Could you check a few things on this model? Use its own coordinates, in mm. Face numbers are marked on the shaded views. A direction names the side the tool comes from. Round coordinates to 2 decimals unless told otherwise and drop trailing zeros. Order: outer loops, then holes, each group sorted by start corner. A loop starts at its lowest first (then second) coordinate and runs counter-clockwise, first axis right, second up. Notation, with made-up numbers: (5, -38.5) - (28, -38.5) arc R23 cw to (28, 0.5) - close; hole circle Ø3 at (-24, 75.25). An arc over 180 degrees is marked (long way). Use one line per item in the form item = value.
from build123d import *

# Parameters (mm, degrees)
TABAN_FLAN_1_DEPTH       = 400
M5_DI_LI_DELIK1_D        = 4.2
IZIM10_R                 = 6
KES_EKSTR_ZYON1_DEPTH    = 451
KENAR_FLAN_1_START       = -100
KENAR_FLAN_1_OUTLINE_W   = 0.163300289
KENAR_FLAN_1_OUTLINE_H   = 2.7366
KENAR_FLAN_1_DEPTH       = 2.7366
KENAR_FLAN_1_START_2     = 97.2634
KENAR_FLAN_1_2_OUTLINE_W = 0.163300289
KENAR_FLAN_1_2_OUTLINE_H = 2.7366
KENAR_FLAN_1_2_DEPTH     = 2.7366
KENAR_FLAN_1_START_3     = -97.2634
KENAR_FLAN_1_3_DEPTH     = 194.5268
KENAR_FLAN_1_4_DEPTH     = 194.5268


# Read off the part's stored shape, not the designer's step: Kenar-Flanş1
# Sheet-metal steps are written as plain solids
with BuildPart() as part:
    # Çizim1 → Taban-Flanş1 (new, symmetric)
    with BuildSketch(Plane(origin=(0, 0, 0), x_dir=(0, 0, -1), z_dir=(1, 0, 0))):
        with BuildLine():
            Line((-100, -50), (-100, -2.7366))
            ThreePointArc((-100, -2.7366), (-99.198468417, -0.801531583), (-97.2634, 0))
            Line((-97.2634, 0), (97.2634, 0))
            ThreePointArc((97.2634, 0), (99.198468417, -0.801531583), (100, -2.7366))
            Line((100, -2.7366), (100, -50))
            Line((100, -50), (98, -50))
            Line((98, -50), (98, -2.7366))
            ThreePointArc((98, -2.7366), (97.784254855, -2.215745145), (97.2634, -2))
            Line((97.2634, -2), (-97.2634, -2))
            ThreePointArc((-97.2634, -2), (-97.784254855, -2.215745145), (-98, -2.7366))
            Line((-98, -2.7366), (-98, -50))
            Line((-98, -50), (-100, -50))
        make_face()
    extrude(amount=TABAN_FLAN_1_DEPTH, both=True)

    # M5 Dişli Delik1 (through all)
    with Locations(Plane(origin=(-385, -15, 100), x_dir=(1, 0, 0), z_dir=(0, 0, 1))):
        with Locations((0, 0), (0, -20)):
            m5_di_li_delik1 = Hole(M5_DI_LI_DELIK1_D / 2)

    # Çizim10 → Kes-Ekstrüzyon1 (cut, through all)
    with BuildSketch(Plane.XY.offset(100)):
        with Locations((-335, -12.5)):
            Circle(IZIM10_R)
        with Locations((-335, -37.5)):
            Circle(IZIM10_R)
    kes_ekstr_zyon1 = extrude(amount=-KES_EKSTR_ZYON1_DEPTH, mode=Mode.SUBTRACT)

    # Aynalama1: M5 Dişli Delik1, Kes-Ekstrüzyon1 across plane
    add(m5_di_li_delik1.mirror(Plane(origin=(0, 0, 0), x_dir=(0, 0, 1), z_dir=(1, 0, 0))), mode=Mode.SUBTRACT)
    add(kes_ekstr_zyon1.mirror(Plane(origin=(0, 0, 0), x_dir=(0, 0, 1), z_dir=(1, 0, 0))), mode=Mode.SUBTRACT)

    # Kenar-Flanş1 outline → Kenar-Flanş1 (cut)
    with BuildSketch(Plane.XY.offset(KENAR_FLAN_1_START)):
        with Locations((399.918349856, -1.3683)):
            Rectangle(KENAR_FLAN_1_OUTLINE_W, KENAR_FLAN_1_OUTLINE_H)
        with Locations((-399.918349856, -1.3683)):
            Rectangle(KENAR_FLAN_1_OUTLINE_W, KENAR_FLAN_1_OUTLINE_H)
    extrude(amount=KENAR_FLAN_1_DEPTH, mode=Mode.SUBTRACT)

    # Kenar-Flan_1 2 outline → Kenar-Flan_1 2 (cut)
    with BuildSketch(Plane.XY.offset(KENAR_FLAN_1_START_2)):
        with Locations((399.918349856, -1.3683)):
            Rectangle(KENAR_FLAN_1_2_OUTLINE_W, KENAR_FLAN_1_2_OUTLINE_H)
        with Locations((-399.918349856, -1.3683)):
            Rectangle(KENAR_FLAN_1_2_OUTLINE_W, KENAR_FLAN_1_2_OUTLINE_H)
    extrude(amount=KENAR_FLAN_1_2_DEPTH, mode=Mode.SUBTRACT)

    # Kenar-Flan_1 3 outline → Kenar-Flan_1 3 (cut)
    with BuildSketch(Plane.XY.offset(KENAR_FLAN_1_START_3)):
        with BuildLine():
            Line((400, 0), (399.836699711, 0))
            ThreePointArc((399.836699711, 0), (399.918386255, -0.001219429), (400, -0.004876629))
            Line((400, -0.004876629), (400, 0))
        make_face()
        with BuildLine():
            ThreePointArc((-400, -0.004876629), (-399.918386255, -0.001219429), (-399.836699711, 0))
            Line((-399.836699711, 0), (-400, 0))
            Line((-400, 0), (-400, -0.004876629))
        make_face()
    extrude(amount=KENAR_FLAN_1_3_DEPTH, mode=Mode.SUBTRACT)

    # Kenar-Flan_1 4 outline → Kenar-Flan_1 4 (add)
    with BuildSketch(Plane.XY.offset(KENAR_FLAN_1_START_3)):
        with BuildLine():
            Line((400, -0.004876629), (400, -2))
            Line((400, -2), (399.836699711, -2))
            ThreePointArc((399.836699711, -2), (399.996129131, -2.017460361), (400.148000323, -2.069013684))
            Line((400.148000323, -2.069013684), (408.661230672, -6.038798191))
            Line((408.661230672, -6.038798191), (409.506467196, -4.226182617))
            Line((409.506467196, -4.226182617), (400.993236847, -0.25639811))
            ThreePointArc((400.993236847, -0.25639811), (400.508494673, -0.083739075), (400, -0.004876629))
        make_face()
        with BuildLine():
            Line((-399.836699711, -2), (-400, -2))
            Line((-400, -2), (-400, -0.004876629))
            ThreePointArc((-400, -0.004876629), (-400.508494673, -0.083739075), (-400.993236847, -0.25639811))
            Line((-400.993236847, -0.25639811), (-409.506467196, -4.226182617))
            Line((-409.506467196, -4.226182617), (-408.661230672, -6.038798191))
            Line((-408.661230672, -6.038798191), (-400.148000323, -2.069013684))
            ThreePointArc((-400.148000323, -2.069013684), (-399.996129131, -2.017460361), (-399.836699711, -2))
        make_face()
    extrude(amount=KENAR_FLAN_1_4_DEPTH)


solid = part.part
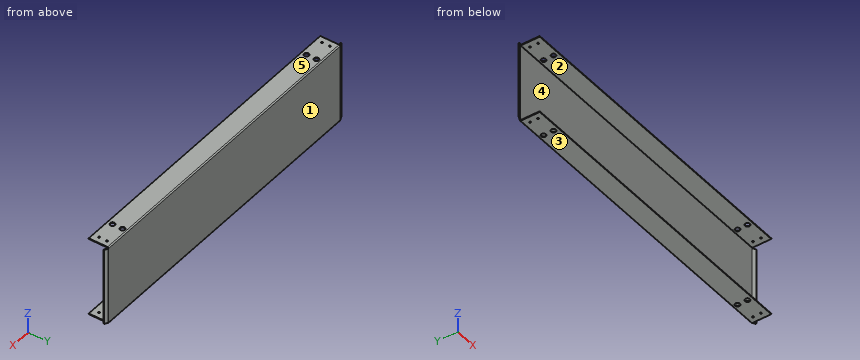
Item 1: Will these pins go through, and if not, where does the flat tip stop? P1, Ø10, axis at y = -6.5, z = -27, coming from the -X side; P2, Ø6, axis at x = 127.5, z = 64, coming from the +Y side; P3, Ø2.5, axis at x = 385, y = -15, coming from the +Z side; P4, Ø1.4, axis at y = -1.5, z = 98.5, coming from the +X side.
Found:
P1 = -409.51
P2 = 0
P3 = through
P4 = 399.84
Item 2: If we mould it in two halves opening along Z, with no side actions, what happens to the marked faces 3, 4 and 5? For each: released by +Z, released by -Z, zero draft, split by the parting line, or undercut.
Found:
face_3 = released by -Z
face_4 = undercut
face_5 = released by +Z
Item 3: I need wall thicknesses on L1, parallel to Z at x = -232, y = -7.5; L2, parallel to Y at x = -385, z = -98.75; L3, parallel to Y at x = -55, z = -27. Which ranges of each line are inside material? Lowest first, please.
Found:
L1 = -100 to -98, 98 to 100
L2 = -50 to -37.1, -32.9 to -17.1, -12.9 to -0.44
L3 = -2 to 0
Item 4: Imagine slicing it at B-B on z = 39. Please give me the cut outline in (x, y), plus the area to 3 significant figures.
Found:
outline = (-409.51, -4.23) - (-408.66, -6.04) - (-400.15, -2.07) arc R0.74 cw to (-399.84, -2) - (399.84, -2) arc R0.74 cw to (400.15, -2.07) - (408.66, -6.04) - (409.51, -4.23) - (400.99, -0.26) arc R2.74 ccw to (399.84, 0) - (-399.84, 0) arc R2.74 ccw to (-400.99, -0.26) - close
area = 1,640 mm2
Item 5: Imagine slicing it at A-A on x = 312. Please give me the cut outline in (y, z).
Found:
outline = (-50, -100) - (-2.74, -100) arc R2.74 ccw to (0, -97.26) - (0, 97.26) arc R2.74 ccw to (-2.74, 100) - (-50, 100) - (-50, 98) - (-2.74, 98) arc R0.74 cw to (-2, 97.26) - (-2, -97.26) arc R0.74 cw to (-2.74, -98) - (-50, -98) - close
Item 6: For the marked faces 1 and 2, which set-ups out of +Z, -Z, +X, -X, +Y, -Y let a thin tool reach every point of the face, with its end or its side?
Found:
face_1 = +Z, -Z, +X, -X, +Y
face_2 = +X, -X, -Y
